The listing builds one solid part. Answer for the finished solid, in the listing's coordinates (mm). A direction names the side the tool comes from. Coordinates: 2 decimals unless noted, no trailing zeros. Order: outer loops, then holes, each group sorted by start corner. A loop starts at its lowest first (then second) coordinate and runs counter-clockwise, first axis right, second up. Notation, with made-up numbers: (-37.75, 78.5) -> (-12.75, 78.5) arc R25 ccw to (-12.75, 96.5) -> close; hole circle Ø5 at (47, 39.25). An arc over 180 degrees is marked (long way). Write each question's results on one line, items separated by ' | '. Start each with the question number.
(1) The part is cut by section B-B, the plane x = -15.5. Give the vertices of the cut face in (y, z).
(2) The part is cut by section C-C, the plane z = -119. Give the vertices of the cut face in (x, y), then the cut area to 3 significant figures.
(3) The part is cut by section A-A, the plane z = -73. Give the vertices of the cut face in (x, y).
(4) Determine the mould class of faces 1 (the face through (-72.196, 2.028, -129.289)), 2 (the face through (50, 2, -36)), 3 (the face through (48.827, 2.028, -101.795)), 4 (the face through (-1, 0, -84)) for opening direction Z: +Z half, -Z half, draft (parallel to the pull), parting line (faces both ways), or undercut.
(5) Given pin 1 (1 mm diameter, centred on x = 46, y = 2.5, fed in from +Z); pin 2 (2 mm diameter, centred on x = -48, y = 2.5, fed in from +Z); pin 3 (4.5 mm diameter, centred on x = 68, z = -125, fed in from +Y), each flat-ended and moving along its own axis, determine where each tip first touches the part or whether it passes through.
(6) A tool of negligible diameter and unlimited length cuts with its end or side. For faces 5 (the face through (-63, 2, -35)), 6 (the face through (58.496, 2.028, -55.944)), from which of +Z, -Z, +X, -X, +Y, -Y can it reach the whole face along a straight path? Write none if from no direction.
(7) The part is cut by section D-D, the plane y = 1. Count the separate pieces of the cut face and the enclosed holes in it, then the cut area to 3 significant figures.
(8) Straight lines are drawn through the part: L1, parallel to X at y = 1.5, z = -125; L2, parallel to X at y = 2.3, z = -63.5; L3, parallel to Z at x = -68, y = 0.95. For each, find the intervals that lie inside material, in ascending order.
```python
from build123d import *

# Parameters (mm, degrees)
BOSS_EXTRUDE1_DEPTH = 4
SKETCH3_R           = 1.7
CUT_EXTRUDE1_DEPTH  = 4
FILLET1_R           = 6
SKETCH4_R           = 1.7
CUT_EXTRUDE2_DEPTH  = 10
CUT_EXTRUDE3_DEPTH  = 10
CHAMFER1_SIZE       = 1.65


with BuildPart() as part:
    # Sketch2 → Boss-Extrude1 (new body)
    with BuildSketch(Plane(origin=(0, 0, 0), x_dir=(1, 0, 0), z_dir=(0, 1, 0))):
        with BuildLine():
            Line((74, 35), (74, 131))
            Line((74, 131), (-74, 131))
            Line((-74, 131), (-74, 35))
            Line((-74, 35), (-58.426149773, 35))
            ThreePointArc((-58.426149773, 35), (-50, 36), (-41.573850227, 35))
            Line((-41.573850227, 35), (41.573850227, 35))
            ThreePointArc((41.573850227, 35), (50, 36), (58.426149773, 35))
            Line((58.426149773, 35), (74, 35))
        make_face()
    extrude(amount=BOSS_EXTRUDE1_DEPTH)

    # Sketch3 → Cut-Extrude1 (cut)
    with BuildSketch(Plane(origin=(0, 4, 0), x_dir=(1, 0, 0), z_dir=(0, 1, 0))):
        with Locations((-66.264045876, -39.264880132)):
            Circle(SKETCH3_R)
        with Locations(Location((-66.264045876, 39.264880132, 0), (0, 0, 270))):
            Circle(SKETCH3_R)
        with Locations(Location((-33.735954124, 39.264880132, 0), (0, 0, 270))):
            Circle(SKETCH3_R)
        with Locations((-10.735119868, 16.264045876)):
            Circle(SKETCH3_R)
        with Locations((-10.735119868, -16.264045876)):
            Circle(SKETCH3_R)
        with Locations((-33.735954124, -39.264880132)):
            Circle(SKETCH3_R)
        with Locations((10.735119868, 16.264045876)):
            Circle(SKETCH3_R)
        with Locations(Location((33.735954124, 39.264880132, 0), (0, 0, 270))):
            Circle(SKETCH3_R)
        with Locations(Location((66.264045876, 39.264880132, 0), (0, 0, 270))):
            Circle(SKETCH3_R)
        with Locations((10.735119868, -16.264045876)):
            Circle(SKETCH3_R)
        with Locations((33.735954124, -39.264880132)):
            Circle(SKETCH3_R)
        with Locations((66.264045876, -39.264880132)):
            Circle(SKETCH3_R)
    extrude(amount=-CUT_EXTRUDE1_DEPTH, mode=Mode.SUBTRACT)

    # Fillet1
    fillet1_edges = [part.edges().sort_by_distance(p)[0] for p in [
        (-74, 2, -131),
        (74, 2, -131),
        (74, 2, -35),
        (-74, 2, -35),
    ]]
    fillet(fillet1_edges, radius=FILLET1_R)

    # Sketch4 → Cut-Extrude2 (cut)
    with BuildSketch(Plane(origin=(0, 4, 0), x_dir=(1, 0, 0), z_dir=(0, 1, 0))):
        with Locations(Location((68, 125, 0), (0, 0, 270))):
            Circle(SKETCH4_R)
        with Locations(Location((-68, 125, 0), (0, 0, 270))):
            Circle(SKETCH4_R)
    extrude(amount=-CUT_EXTRUDE2_DEPTH, mode=Mode.SUBTRACT)

    # Sketch5 → Cut-Extrude3 (cut)
    with BuildSketch(Plane(origin=(0, 4, 0), x_dir=(1, 0, 0), z_dir=(0, 1, 0))):
        with BuildLine():
            Line((-12.5, 121), (-28.674783736, 121))
            ThreePointArc((-28.674783736, 121), (-36.777367456, 116.860728372), (-38.172192195, 107.86962741))
            Line((-38.172192195, 107.86962741), (-22.851640419, 61.387768193))
            ThreePointArc((-22.851640419, 61.387768193), (-19.214960332, 56.415557063), (-13.35423196, 54.518140784))
            Line((-13.35423196, 54.518140784), (-12.5, 54.518140784))
            ThreePointArc((-12.5, 54.518140784), (-5.428932188, 57.447072972), (-2.5, 64.518140784))
            Line((-2.5, 64.518140784), (-2.5, 111))
            ThreePointArc((-2.5, 111), (-5.428932188, 118.071067812), (-12.5, 121))
        make_face()
        with BuildLine():
            Line((-60, 59.518140784), (-60, 97.798571602))
            ThreePointArc((-60, 97.798571602), (-58.535533906, 101.334105508), (-55, 102.798571602))
            Line((-55, 102.798571602), (-51.831780224, 102.798571602))
            ThreePointArc((-51.831780224, 102.798571602), (-48.790398959, 101.767198569), (-47.003737142, 99.098571602))
            Line((-47.003737142, 99.098571602), (-36.696339461, 60.818140784))
            ThreePointArc((-36.696339461, 60.818140784), (-37.555755576, 56.476759519), (-41.524382543, 54.518140784))
            Line((-41.524382543, 54.518140784), (-55, 54.518140784))
            ThreePointArc((-55, 54.518140784), (-58.535533906, 55.982606878), (-60, 59.518140784))
        make_face()
    cut_extrude3 = extrude(amount=-CUT_EXTRUDE3_DEPTH, mode=Mode.SUBTRACT)

    # Mirror1: Cut-Extrude3 across plane
    add(cut_extrude3.mirror(Plane(origin=(0, 0, 0), x_dir=(0, 0, 1), z_dir=(1, 0, 0))), mode=Mode.SUBTRACT)

    # Chamfer1
    chamfer1_edges = [part.edges().sort_by_distance(p)[0] for p in [
        (-68, 4, -126.7),
        (68, 4, -126.7),
    ]]
    chamfer(chamfer1_edges, length=CHAMFER1_SIZE)


solid = part.part
```
Established:
1) outline: (0, -131) -> (4, -131) -> (4, -121) -> (0, -121) -> close; (0, -54.75) -> (4, -54.75) -> (4, -35) -> (0, -35) -> close
2) outline: (-74, 0) -> (-34.67, 0) -> (-34.67, 4) -> (-74, 4) -> close; (-6.5, 0) -> (6.5, 0) -> (6.5, 4) -> (-6.5, 4) -> close; (34.67, 0) -> (74, 0) -> (74, 4) -> (34.67, 4) -> close | area: 367 mm^2
3) outline: (-74, 0) -> (-60, 0) -> (-60, 4) -> (-74, 4) -> close; (-39.98, 0) -> (-26.68, 0) -> (-26.68, 4) -> (-39.98, 4) -> close; (-2.5, 0) -> (2.5, 0) -> (2.5, 4) -> (-2.5, 4) -> close; (26.68, 0) -> (39.98, 0) -> (39.98, 4) -> (26.68, 4) -> close; (60, 0) -> (74, 0) -> (74, 4) -> (60, 4) -> close
4) face 1: -Z half | face 2: +Z half | face 3: undercut | face 4: draft
5) pin 1: stops at z = -35.72 | pin 2: stops at z = -35.87 | pin 3: stops at y = 2.9
6) face 5: +Z, +X, -X, +Y, -Y | face 6: +Y, -Y
7) separate pieces: 1 | enclosed holes: 10 | area: 8,690 mm^2
8) L1: x = -74 to -69.7, -66.3 to 66.3, 69.7 to 74 | L2: x = -74 to -60, -37.42 to -23.55, -2.55 to 2.55, 23.55 to 37.42, 60 to 74 | L3: z = -131 to -126.7, -123.3 to -35
